Geometry check sheet. Reference: the model listing, model coordinates, mm. A direction names the side the tool comes from. Give positions to 0.01 mm unless a question says otherwise; leave off trailing zeros. Write each loop counter-clockwise with the first axis right and the second up, starting at its lowest first coordinate (ties: lowest second). Pieces come first, ordered by that corner, then holes. Notation, with made-up numbers: M 0,76.25 L 18,76.25 A25 ccw 18,103.25 Z; hole C -4.5,51 d6. An arc over 180 degrees is marked long. Write each question's results on one line, items separated by ' | '.
```python
from build123d import *

# Parameters (mm, degrees)
PAD001_DEPTH = 4
PAD_DEPTH    = 6
SKETCH002_R  = 3.5
PAD002_DEPTH = 3


with BuildPart() as groove_pad:
    # Sketch001 → Pad001 (new body)
    with BuildSketch(Plane.XY.offset(2)):
        with BuildLine():
            ThreePointArc((-4, -64.360473), (-7.470504, -66.562647), (-9.878753, -69.893457))
            Line((-13.664632, -78.012293), (-9.878753, -69.893457))
            ThreePointArc((-13.664632, -78.012293), (-12.699944, -78.175133), (-11.733319, -78.326044))
            ThreePointArc((-12.266666, -81.886317), (-10.219864, -80.372853), (-11.733319, -78.326044))
            ThreePointArc((-15.237734, -81.385819), (-13.754477, -81.649583), (-12.266666, -81.886317))
            Line((-16.45811, -84.00292), (-15.237734, -81.385819))
            ThreePointArc((-16.45811, -84.00292), (0, -85.6), (16.45811, -84.00292))
            Line((16.45811, -84.00292), (15.237734, -81.385819))
            ThreePointArc((12.266666, -81.886317), (13.754477, -81.649583), (15.237734, -81.385819))
            ThreePointArc((11.733319, -78.326044), (10.219864, -80.372853), (12.266666, -81.886317))
            ThreePointArc((11.733319, -78.326044), (12.699944, -78.175133), (13.664632, -78.012293))
            Line((9.878753, -69.893457), (13.664632, -78.012293))
            ThreePointArc((9.878753, -69.893457), (7.470504, -66.562647), (4, -64.360473))
            Line((4, -61.187975), (4, -64.360473))
            ThreePointArc((4, -61.187975), (0, -60.6), (-4, -61.187975))
            Line((-4, -64.360473), (-4, -61.187975))
        make_face()
    extrude(amount=PAD001_DEPTH)


with BuildPart() as groove_cut:
    # Sketch → Pad (new body)
    with BuildSketch(Plane.XY):
        with BuildLine():
            ThreePointArc((-18.036325, -82.655012), (0, -84.6), (18.036325, -82.655012))
            Line((18.036325, -82.655012), (11.691387, -69.048259))
            ThreePointArc((11.691387, -69.048259), (0, -61.6), (-11.691387, -69.048259))
            Line((-18.036325, -82.655012), (-11.691387, -69.048259))
        make_face()
    extrude(amount=PAD_DEPTH)

    # Cut: cut Groove_Pad
    add(groove_pad.part, mode=Mode.SUBTRACT)


with BuildPart() as fusion:
    # Sketch002 → Pad002 (new body)
    with BuildSketch(Plane.XY):
        with Locations((0, -74.5)):
            Circle(SKETCH002_R)
    extrude(amount=PAD002_DEPTH)

    # Fusion: union Groove_Cut
    add(groove_cut.part)


solid = fusion.part
```
Q1. Section check D-D (z = 1.55). Enter the section's corners in (x, y).
Answer key:
outline: M -18.04,-82.66 A84.6 ccw 18.04,-82.66 L 11.69,-69.05 A12.9 ccw -11.69,-69.05 Z
Q2. Section check B-B (x = 0). Enter the section's corners in (y, z).
Answer key:
outline: M -84.6,0 L -61.6,0 L -61.6,2 L -71,2 L -71,3 L -78,3 L -78,2 L -84.6,2 Z
Q3. Section check A-A (z = 3.4). Enter the section's corners in (x, y).
Answer key:
outline: M -18.04,-82.66 A84.6 ccw -16.02,-83.07 L -15.24,-81.39 A82.8 ccw -12.27,-81.89 A1.8 ccw -11.73,-78.33 A79.2 cw -13.66,-78.01 L -9.88,-69.89 A10.9 cw -4,-64.36 L -4,-62.24 A12.9 ccw -11.69,-69.05 Z; M 4,-64.36 A10.9 cw 9.88,-69.89 L 13.66,-78.01 A79.2 cw 11.73,-78.33 A1.8 ccw 12.27,-81.89 A82.8 ccw 15.24,-81.39 L 16.02,-83.07 A84.6 ccw 18.04,-82.66 L 11.69,-69.05 A12.9 ccw 4,-62.24 Z
Q4. Section check C-C (y = -63). Enter the section's corners in (x, z), then the cut area to 3 significant figures.
Answer key:
outline: M -5.84,0 L 5.84,0 L 5.84,6 L 4,6 L 4,2 L -4,2 L -4,6 L -5.84,6 Z | area: 38.1 mm2
Q5. Depth check by flat-ended pin: P1, Ø4, axis at x = -2, y = -80.5, coming from the +Z side; P2, Ø2.5, axis at y = -63.5, z = 4.5, coming from the -X side; P3, Ø1.1, axis at y = -63, z = 4, coming from the +X side. Enter the tip coordinate at first touch or a pass-through.
Answer key:
P1: stops at z = 2 | P2: stops at x = -8.45 | P3: stops at x = 6.82
Q6. Access from +Z, -Z, +X, -X, +Y, -Y to the whole of each face (thin tool, end or side, straight path). Record for faces 4 (the face through (0, -75, 0)), 5 (the face through (0, -74, 3)), 6 (the face through (-7.428, -66.523, 3.972)), 7 (the face through (11.745, -73.896, 3.972)).
Answer key:
face 4: -Z, +X, -X, +Y, -Y | face 5: +Z, +Y, -Y | face 6: +Z, -Y | face 7: +Z
Q7. Material ranges on probe 1 along Z at (x, y) = (-7.5, -76.75); probe 2 along X at (y, z) = (-67.5, 3.05); probe 3 along X at (y, z) = (-64.5, 2.15), recorded low to high. Write a range as [from, to].
Answer key:
probe 1: z = [0, 2] | probe 2: x = [-10.84, -8.36], [8.36, 10.84] | probe 3: x = [-8.15, -4.34], [4.34, 8.15]
Q8. Release check for a two-part mould opening along X. For faces 1 (the face through (-4.29, -84.49, 1.62)), 2 (the face through (-12.713, -78.173, 3.972)), 3 (the face through (14.91, -75.95, 2.96)) record: released by +X, released by -X, zero draft, split by the parting line, or undercut.
Answer key:
face 1: split by the parting line | face 2: undercut | face 3: released by +X
